For this review, take the finished solid that the model builds, in its own axes (mm). A direction names the side the tool comes from. Coordinates: 2 decimals unless noted, no trailing zeros. Order: outer loops, then holes, each group sorted by start corner. A loop starts at its lowest first (then second) coordinate and runs counter-clockwise, first axis right, second up. Notation, with made-up numbers: (45.5, 43) -> (79.5, 43) arc R13 cw to (79.5, 58) -> close; hole circle Ø3 at (-3, -19.5). An arc over 180 degrees is marked (long way). Write item = value, one per line. Start each with the question number.
1) Wall thickness on probe 1 along Y at (x, z) = (0, 28); probe 2 along X at (y, z) = (7, 31.5); probe 3 along Y at (x, z) = (0, 8): over which ranges is each line inside the solid? List them lowest first. Write a range as [from, to].
2) Draft analysis for pull direction X (two halves, no side actions). For faces 1 (the face through (-5.25, -18, 31)), 2 (the face through (-2, -17.5, 33)), 3 (the face through (4.75, -18, 31)), 4 (the face through (13.61, -6.04, 11.83)), state which applies: +X half, -X half, draft (parallel to the pull), parting line (faces both ways), or undercut.
3) Consider section D-D on z = 22.5. Give the boundary of the cut face in (x, y), and give its area (3 significant figures).
4) Consider section C-C on x = 11. Give the boundary of the cut face in (y, z).
5) Consider section B-B on x = 0.5. Give the boundary of the cut face in (y, z).
6) Insertion check: pin 1 Ø5 at (y, z) = (-5.5, 29.5) entering from -X; pin 2 Ø1 at (x, z) = (6, 19) entering from -Y (3 decimals); pin 3 Ø3 at (x, z) = (7, 7) entering from +Y. Each pin has a flat end and moves straight along its axis. Give the tip position at first contact, or say it passes through.
7) Consider section A-A on y = 8.5. Give the boundary of the cut face in (x, z), and give its area (3 significant figures).
8) Machinability: for faces 5 (the face through (-3.2, -15.4, 33.3)), 6 (the face through (-13.571, -6.065, 11.832)), 7 (the face through (0, -21, 30)), 8 (the face through (-0.38, -19.23, 30.17)), which of the approach directions +Z, -Z, +X, -X, +Y, -Y give a long, thin tool a straight path to every point of the face, cutting with its end or side? Answer none if there is none.
from build123d import *

# Parameters (mm, degrees)
SKETCH1_R                = 16
BOSS_EXTRUDE1_DEPTH      = 36
SKETCH4_R                = 13.9
CUT_EXTRUDE1_DEPTH       = 43.520583251
CUT_EXTRUDE3_DEPTH       = 43.520583251
CUT_EXTRUDE3_DEPTH_BACK  = 43.520583251
BOSS_EXTRUDE2_REACH      = 56.046
BOSS_EXTRUDE2_END_RADIUS = 16
SKETCH8_W                = 10
SKETCH8_H                = 8
SKETCH7_R                = 1.7
CUT_EXTRUDE4_DEPTH       = 25
SKETCH10_R               = 3.1
CUT_EXTRUDE6_DEPTH       = 17.5
CUT_EXTRUDE7_DEPTH       = 24


with BuildPart() as part:
    # Sketch1 → Boss-Extrude1 (new body)
    with BuildSketch(Plane.XY):
        Circle(SKETCH1_R)
    extrude(amount=BOSS_EXTRUDE1_DEPTH)

    # Sketch4 → Cut-Extrude1 (cut, through all)
    with BuildSketch(Plane(origin=(0, 0, 0), x_dir=(-1, 0, 0), z_dir=(0, 0, -1))):
        Circle(SKETCH4_R)
    extrude(amount=-CUT_EXTRUDE1_DEPTH, mode=Mode.SUBTRACT)

    # Sketch6 → Cut-Extrude3 (cut, two sides: drawn at the far end of the back side and taken through both)
    with BuildSketch(Plane(origin=(0, 0, 0), x_dir=(0, 0, -1), z_dir=(1, 0, 0)).offset(-CUT_EXTRUDE3_DEPTH_BACK)):
        Polygon((-36, 16), (-32.636664471, 16), (-36, -16), align=None)
    extrude(amount=CUT_EXTRUDE3_DEPTH + CUT_EXTRUDE3_DEPTH_BACK, mode=Mode.SUBTRACT)

    # Boss-Extrude2: up to this cylinder (the profile starts outside it)
    boss_extrude2_end = Plane(origin=(0, 0, 31), z_dir=(0, 0, -1)) * Cylinder(BOSS_EXTRUDE2_END_RADIUS, 145.092, mode=Mode.PRIVATE)
    # Sketch8 → Boss-Extrude2 (add, up to the surface)
    with BuildSketch(Plane(origin=(0, -21, 0), x_dir=(1, 0, 0), z_dir=(0, 1, 0)), mode=Mode.PRIVATE) as boss_extrude2_sk1:
        with Locations((-0.25, -31)):
            Rectangle(SKETCH8_W, SKETCH8_H)
    boss_extrude2_tool1 = extrude(boss_extrude2_sk1.sketch, amount=BOSS_EXTRUDE2_REACH, mode=Mode.PRIVATE) - boss_extrude2_end
    add(boss_extrude2_tool1.solids().sort_by_distance((-0.25, -21, 31))[0])

    # Sketch7 → Cut-Extrude4 (cut)
    with BuildSketch(Plane(origin=(0, 0, 0), x_dir=(1, 0, 0), z_dir=(0, 1, 0))):
        with Locations(Location((-0.45, -31.867848556, 0), (0, 0, 270))):
            Circle(SKETCH7_R)
    extrude(amount=-CUT_EXTRUDE4_DEPTH, mode=Mode.SUBTRACT)

    # Sketch10 → Cut-Extrude6 (cut)
    with BuildSketch(Plane(origin=(0, 0, 0), x_dir=(1, 0, 0), z_dir=(0, 1, 0))):
        with Locations(Location((-0.45, -31.867848556, 0), (0, 0, 270))):
            Circle(SKETCH10_R)
    extrude(amount=-CUT_EXTRUDE6_DEPTH, mode=Mode.SUBTRACT)

    # Sketch11 → Cut-Extrude7 (cut)
    with BuildSketch(Plane(origin=(0, 0, 0), x_dir=(-1, 0, 0), z_dir=(0, 0, -1))):
        Polygon((-51.788319146, 16), (0, -13.9), (51.788319146, 16), align=None)
    extrude(amount=-CUT_EXTRUDE7_DEPTH, mode=Mode.SUBTRACT)


solid = part.part
Answer sheet:
q1.probe_1 = [-21, -13.9], [13.9, 16]
q1.probe_2 = [-14.39, -12.01], [12.01, 14.39]
q1.probe_3 = [-16, -13.9]
q2.face_1 = -X half
q2.face_2 = undercut
q2.face_3 = +X half
q2.face_4 = undercut
q3.outline = (-15.15, -5.15) arc R16 ccw to (15.15, -5.15) -> (12.04, -6.95) arc R13.9 cw to (-12.04, -6.95) -> close
q3.area = 72.6 mm2
q4.outline = (-11.62, 0) -> (-8.5, 0) -> (-8.5, 35.21) -> (-11.62, 35.54) -> close; (8.5, 24) -> (11.62, 24) -> (11.62, 33.1) -> (8.5, 33.43) -> close
q5.outline = (-21, 27) -> (-15.99, 27) -> (-15.99, 0) -> (-13.89, 0) -> (-13.89, 28.92) -> (-17.5, 28.92) -> (-17.5, 30.46) -> (-21, 30.46) -> close; (-21, 33.28) -> (-17.5, 33.28) -> (-17.5, 34.82) -> (-13.89, 34.82) -> (-13.89, 35.78) -> (-15.99, 36) -> (-15.99, 35) -> (-21, 35) -> close; (13.89, 24) -> (15.99, 24) -> (15.99, 32.64) -> (13.89, 32.86) -> close
q6.pin_1 = -15.72
q6.pin_2 = -15.025
q6.pin_3 = -11
q7.outline = (-13.56, 24) -> (-11, 24) -> (-11, 33.42) -> (-13.56, 33.42) -> close; (11, 24) -> (13.56, 24) -> (13.56, 33.42) -> (11, 33.42) -> close
q7.area = 48.2 mm2
q8.face_5 = none
q8.face_6 = -Z, +Y
q8.face_7 = +Z, -Z, +X, -X, -Y
q8.face_8 = -Y
